Geometry check sheet. Reference: the model listing, model coordinates, mm. Face numbers are marked on the shaded views. A direction names the side the tool comes from. Coordinates: 2 decimals unless noted, no trailing zeros. Write each loop counter-clockwise with the first axis right and the second up, starting at its lowest first coordinate (ties: lowest second). Pieces come first, ordered by that corner, then holes. Notation, with made-up numbers: (64.25, 24.25) -> (123.25, 24.25) arc R18 ccw to (123.25, 31.25) -> close; hole circle Ø6 at (73.25, 38). An arc over 180 degrees is marked (long way). Put each result on its own line as item: value. Start each with the question number.
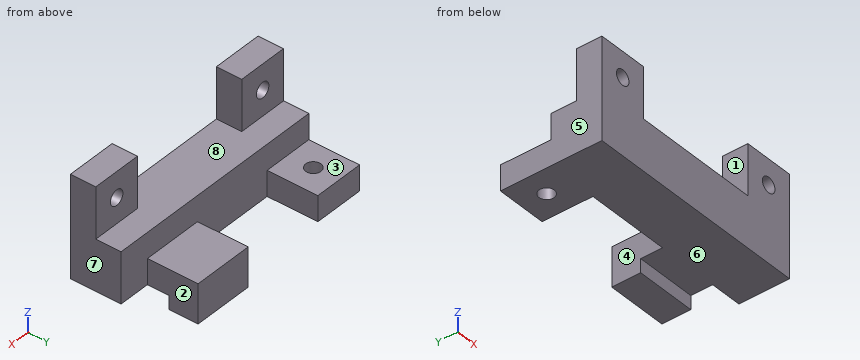
from build123d import *

# Parameters (mm, degrees)
SKETCH1_W           = 45
SKETCH1_H           = 10
BOSS_EXTRUDE1_DEPTH = 10
SKETCH2_W           = 10
SKETCH2_H           = 5
SKETCH2_W_2         = 12
BOSS_EXTRUDE2_DEPTH = 10
SKETCH3_W           = 10
SKETCH3_H           = 5
BOSS_EXTRUDE3_DEPTH = 10
SKETCH4_R           = 1.5
CUT_EXTRUDE1_DEPTH  = 5
SKETCH9_R           = 1.5
CUT_EXTRUDE6_DEPTH  = 5
SKETCH10_R          = 1.5
CUT_EXTRUDE7_DEPTH  = 5
SKETCH11_W          = 12
SKETCH11_H          = 5.7
BOSS_EXTRUDE4_DEPTH = 2.7
SKETCH7_W           = 10
SKETCH7_H           = 10
BOSS_EXTRUDE5_DEPTH = 35
SKETCH13_W          = 12
SKETCH13_H          = 5
BOSS_EXTRUDE6_DEPTH = 10
SKETCH14_W          = 12
SKETCH14_H          = 5.7
BOSS_EXTRUDE7_DEPTH = 2.7
SKETCH15_W          = 5
SKETCH15_H          = 10
CUT_EXTRUDE9_DEPTH  = 50
SKETCH16_W          = 10
SKETCH16_H          = 5
BOSS_EXTRUDE8_DEPTH = 10
SKETCH17_R          = 1.5
CUT_EXTRUDE10_DEPTH = 5


with BuildPart() as part:
    # Sketch1 → Boss-Extrude1 (new body)
    with BuildSketch(Plane.XY):
        with Locations((22.5, 5)):
            Rectangle(SKETCH1_W, SKETCH1_H)
    extrude(amount=BOSS_EXTRUDE1_DEPTH)

    # Sketch2 → Boss-Extrude2 (add)
    with BuildSketch(Plane(origin=(0, 10, 0), x_dir=(1, 0, 0), z_dir=(0, 1, 0))):
        with Locations((40, -2.5)):
            Rectangle(SKETCH2_W, SKETCH2_H)
        with Locations((12.3, -2.5)):
            Rectangle(SKETCH2_W_2, SKETCH2_H)
    extrude(amount=BOSS_EXTRUDE2_DEPTH)

    # Sketch3 → Boss-Extrude3 (add)
    with BuildSketch(Plane.XY.offset(10)):
        with Locations((5, 2.5)):
            Rectangle(SKETCH3_W, SKETCH3_H)
        with Locations((40, 2.5)):
            Rectangle(SKETCH3_W, SKETCH3_H)
    extrude(amount=BOSS_EXTRUDE3_DEPTH)

    # Sketch4 → Cut-Extrude1 (cut)
    with BuildSketch(Plane.ZY):
        with Locations((5, 5)):
            Circle(SKETCH4_R)
    extrude(amount=-CUT_EXTRUDE1_DEPTH, mode=Mode.SUBTRACT)

    # Sketch9 → Cut-Extrude6 (cut)
    with BuildSketch(Plane(origin=(0, 5, 0), x_dir=(1, 0, 0), z_dir=(0, 1, 0))):
        with Locations(Location((40, -15, 0), (0, 0, 180))):
            Circle(SKETCH9_R)
    extrude(amount=-CUT_EXTRUDE6_DEPTH, mode=Mode.SUBTRACT)

    # Sketch10 → Cut-Extrude7 (cut)
    with BuildSketch(Plane.XY.offset(5)):
        with Locations((40, 15)):
            Circle(SKETCH10_R)
    extrude(amount=-CUT_EXTRUDE7_DEPTH, mode=Mode.SUBTRACT)

    # Sketch11 → Boss-Extrude4 (add)
    with BuildSketch(Plane(origin=(0, 0, 0), x_dir=(-1, 0, 0), z_dir=(0, 0, -1))):
        with Locations((-12.3, 17.15)):
            Rectangle(SKETCH11_W, SKETCH11_H)
    extrude(amount=BOSS_EXTRUDE4_DEPTH)

    # Sketch7 → Boss-Extrude5 (add)
    with BuildSketch(Plane(origin=(45, 0, 0), x_dir=(0, 0, -1), z_dir=(1, 0, 0))):
        with Locations((-5, 5)):
            Rectangle(SKETCH7_W, SKETCH7_H)
    extrude(amount=BOSS_EXTRUDE5_DEPTH)

    # Sketch13 → Boss-Extrude6 (add)
    with BuildSketch(Plane(origin=(0, 10, 0), x_dir=(1, 0, 0), z_dir=(0, 1, 0))):
        with Locations((67.7, -2.5)):
            Rectangle(SKETCH13_W, SKETCH13_H)
    extrude(amount=BOSS_EXTRUDE6_DEPTH)

    # Sketch14 → Boss-Extrude7 (add)
    with BuildSketch(Plane(origin=(0, 0, 0), x_dir=(-1, 0, 0), z_dir=(0, 0, -1))):
        with Locations((-67.7, 17.15)):
            Rectangle(SKETCH14_W, SKETCH14_H)
    extrude(amount=BOSS_EXTRUDE7_DEPTH)

    # Sketch15 → Cut-Extrude9 (cut)
    with BuildSketch(Plane.ZY.offset(-35)):
        Polygon((20, 20), (5, 20), (5, 10), (0, 10), (0, 0), (20, 0), align=None)
        with Locations((2.5, 15)):
            Rectangle(SKETCH15_W, SKETCH15_H)
        Polygon((0, 10), (0, 20), (-5, 20), (-5, 0), (0, 0), align=None)
    extrude(amount=CUT_EXTRUDE9_DEPTH, mode=Mode.SUBTRACT)

    # Sketch16 → Boss-Extrude8 (add)
    with BuildSketch(Plane.XY.offset(10)):
        with Locations((75, 2.5)):
            Rectangle(SKETCH16_W, SKETCH16_H)
    extrude(amount=BOSS_EXTRUDE8_DEPTH)

    # Sketch17 → Cut-Extrude10 (cut)
    with BuildSketch(Plane(origin=(0, 5, 0), x_dir=(1, 0, 0), z_dir=(0, 1, 0))):
        with Locations(Location((75, -15, 0), (0, 0, 180))):
            Circle(SKETCH17_R)
    extrude(amount=-CUT_EXTRUDE10_DEPTH, mode=Mode.SUBTRACT)


solid = part.part
Item 1: Access from +Z, -Z, +X, -X, +Y, -Y to the whole of each face (thin tool, end or side, straight path). Record for the marked faces 1, 2, 3 and 4.
Item 2: Section check B-B, the plane x = 40. Enter the section's corners in (y, z).
Item 3: Mould release check, pull along X, two halves, no side actions. Record for the marked faces 5, 6, 7 and 8: released by +X, released by -X, zero draft, split by the parting line, or undercut.
Item 4: Section check D-D, the plane y = 10.75. Enter the section's corners in (x, z), and give its area (3 significant figures).
Item 5: Go/stop test with flat-tipped pins: P1, Ø4, axis at x = 40, y = 15, coming from the +Z side; P2, Ø6, axis at y = 15, z = 0, coming from the +X side; P3, Ø3, axis at x = 65.5, z = -2, coming from the -Y side; P4, Ø2.5, axis at x = 75, z = 15, coming from the +Y side. Record where each tip stops, or that it passes through.
Item 6: Section check A-A, the plane z = 15. Enter the section's corners in (x, y), and give its area (3 significant figures).
Item 7: Scan lines: line 1 along X through (y, z) = (12, 3); line 2 along X through (y, z) = (3, 18.5); line 3 along Z through (x, y) = (40, 2.3). Record each from-to range of solid material in increasing order. Write a range as [from, to].
Item 8: Section check C-C, the plane z = 12.5. Enter the section's corners in (x, y).
From the geometry:
1. face 1: +Z, +Y, -Y
1. face 2: +Z, -Z, +X, +Y
1. face 3: +Z, +X, -X, +Y
1. face 4: +Z, -Z, +Y
2. outline: (0, 0) -> (13.5, 0) -> (13.5, 5) -> (10, 5) -> (10, 10) -> (5, 10) -> (5, 13.5) -> (0, 13.5) -> close; (0, 16.5) -> (5, 16.5) -> (5, 20) -> (0, 20) -> close; (16.5, 0) -> (20, 0) -> (20, 5) -> (16.5, 5) -> close
3. face 5: released by -X
3. face 6: zero draft
3. face 7: released by +X
3. face 8: undercut
4. outline: (35, 0) -> (45, 0) -> (45, 5) -> (35, 5) -> close; (61.7, 0) -> (73.7, 0) -> (73.7, 5) -> (61.7, 5) -> close
4. area: 110 mm²
5. P1: z = 5
5. P2: x = 73.7
5. P3: y = 14.3
5. P4: through
6. outline: (35, 0) -> (38.5, 0) -> (38.5, 5) -> (35, 5) -> close; (41.5, 0) -> (45, 0) -> (45, 5) -> (41.5, 5) -> close; (70, 0) -> (73.5, 0) -> (73.5, 5) -> (70, 5) -> close; (76.5, 0) -> (80, 0) -> (80, 5) -> (76.5, 5) -> close
6. area: 70.0 mm²
7. line 1: [35, 45], [61.7, 73.7]
7. line 2: [35, 45], [70, 80]
7. line 3: [0, 13.5], [16.5, 20]
8. outline: (35, 0) -> (45, 0) -> (45, 5) -> (35, 5) -> close; (70, 0) -> (80, 0) -> (80, 5) -> (70, 5) -> close
